Geometry check sheet. Reference: the model listing, model coordinates, mm. Face numbers are marked on the shaded views. A direction names the side the tool comes from. Give positions to 0.01 mm unless a question says otherwise; leave off trailing zeros. Write each loop counter-clockwise with the first axis right and the second up, starting at its lowest first coordinate (ties: lowest second). Pieces come first, ordered by that corner, then holes. Notation, with made-up numbers: M 58.25,74.25 L 62.25,74.25 A26 cw 62.25,102.25 Z; hole C 62.5,27 d6. An arc over 180 degrees is marked long. One line per item, written item: value. Start each with the question number.
1. Cross-section at B-B on x = 1.75. Record the cut outline in (y, z), then the cut area to 3 significant figures.
2. Gauge pin test, flat ends, axial feed: pin 1 (1.6 mm diameter, centred on x = -9, z = 4, fed in from +Y); pin 2 (4 mm diameter, centred on x = 9, y = -7, fed in from +Z); pin 3 (2 mm diameter, centred on x = 0, z = 21, fed in from +Y). Record the tip position at first contact, or that the pin passes through.
3. Tool access check on the marked faces 4, 5 and 6. Record the directions out of +Z, -Z, +X, -X, +Y, -Y that give a thin tool (end or side, any length) a straight path to the whole face; none if there is none.
4. Cross-section at C-C on y = -4. Record the cut outline in (x, z).
5. Scan lines: line 1 (Y direction, x = 0, z = 1.4); line 2 (X direction, y = -5, z = 8.5); line 3 (Y direction, x = 4.25, z = 15.5). Record each from-to range of solid material in increasing order.
6. Release check for a two-part mould opening along X. For the marked faces 1, 2 and 3 record: pulls with the +X half, pulls with the -X half, needs draft (parallel to the pull), parting line crosses it, or undercut.
7. Cross-section at A-A on z = 9. Record the cut outline in (x, y).
8. Cross-section at D-D on z = 4. Count the separate pieces of the cut face and the enclosed holes in it, then the cut area to 3 significant figures.
from build123d import *

# Parameters (mm, degrees)
BOSS_EXTRUDE1_DEPTH = 3
SKETCH2_W           = 13
SKETCH2_H           = 15
BOSS_EXTRUDE2_DEPTH = 27.5
SKETCH3_W           = 10.6
SKETCH3_H           = 13
CUT_EXTRUDE1_DEPTH  = 26.5
CUT_EXTRUDE2_DEPTH  = 31.5
SKETCH5_W           = 1.5
SKETCH5_H           = 27.57988307
CUT_EXTRUDE3_DEPTH  = 4
BOSS_EXTRUDE4_DEPTH = 2
FILLET2_R           = 1.5
FILLET3_R           = 1.5
SKETCH7_R           = 1
CUT_EXTRUDE4_DEPTH  = 4


with BuildPart() as part:
    # Sketch1 → Boss-Extrude1 (new body)
    with BuildSketch(Plane.XY):
        with BuildLine():
            Line((8.035256759, -13.057292233), (-7.964743241, -13.057292233))
            Line((-7.964743241, -13.057292233), (-7.964743241, 12.942707767))
            ThreePointArc((-7.964743241, 12.942707767), (-0.020633322, 16.942707767), (8.035256759, 13.172891138))
            Line((8.035256759, 13.172891138), (8.035256759, -13.057292233))
        make_face()
    extrude(amount=BOSS_EXTRUDE1_DEPTH)

    # Sketch2 → Boss-Extrude2 (add)
    with BuildSketch(Plane.XY.offset(3)):
        with Locations((0.035256759, -5.557292233)):
            Rectangle(SKETCH2_W, SKETCH2_H)
    extrude(amount=BOSS_EXTRUDE2_DEPTH)

    # Sketch3 → Cut-Extrude1 (cut, symmetric)
    with BuildSketch(Plane.XY.offset(3)):
        with Locations((-0.014743241, -5.807292233)):
            Rectangle(SKETCH3_W, SKETCH3_H)
    extrude(amount=CUT_EXTRUDE1_DEPTH, both=True, mode=Mode.SUBTRACT)

    # Sketch4 → Cut-Extrude2 (cut, through all)
    with BuildSketch(Plane.XY.offset(30.5)):
        with BuildLine():
            Line((-2.5, -8.94154935), (-2.5, -2.55973464))
            ThreePointArc((-2.5, -2.55973464), (0, -0.05973464), (2.5, -2.55973464))
            Line((2.5, -2.55973464), (2.5, -8.94154935))
            ThreePointArc((2.5, -8.94154935), (0, -11.44154935), (-2.5, -8.94154935))
        make_face()
    extrude(amount=-CUT_EXTRUDE2_DEPTH, mode=Mode.SUBTRACT)

    # Sketch5 → Cut-Extrude3 (cut, through all)
    with BuildSketch(Plane.XY.offset(3)):
        with Locations((-7.214743241, 0.732649302)):
            Rectangle(SKETCH5_W, SKETCH5_H)
        with Locations((7.285256759, 0.732649302)):
            Rectangle(SKETCH5_W, SKETCH5_H)
    extrude(amount=-CUT_EXTRUDE3_DEPTH, mode=Mode.SUBTRACT)

    # Sketch6 → Boss-Extrude4 (add)
    with BuildSketch(Plane.XY.offset(3)):
        Polygon((-6.464743241, -3.398686813), (-9.964743241, -3.398686813), (-9.964743241, -7.898686813), (-6.464743241, -7.898686813), (-6.464743241, -9.398686813), (-11.464743241, -9.398686813), (-11.464743241, -1.898686813), (-6.464743241, -1.898686813), align=None)
        Polygon((6.535256759, -3.398686813), (6.535256759, -1.898686813), (11.535256759, -1.898686813), (11.535256759, -9.398686813), (6.535256759, -9.398686813), (6.535256759, -7.898686813), (10.035256759, -7.898686813), (10.035256759, -3.398686813), align=None)
    extrude(amount=BOSS_EXTRUDE4_DEPTH)

    # Fillet2
    fillet2_edges = [part.edges().sort_by_distance(p)[0] for p in [
        (-9.964743241, -3.398686813, 4),
        (-11.464743241, -1.898686813, 4),
        (-11.464743241, -9.398686813, 4),
        (-9.964743241, -7.898686813, 4),
    ]]
    fillet(fillet2_edges, radius=FILLET2_R)

    # Fillet3
    fillet3_edges = [part.edges().sort_by_distance(p)[0] for p in [
        (10.035256759, -3.398686813, 4),
        (10.035256759, -7.898686813, 4),
        (11.535256759, -9.398686813, 4),
        (11.535256759, -1.898686813, 4),
    ]]
    fillet(fillet3_edges, radius=FILLET3_R)

    # Sketch7 → Cut-Extrude4 (cut, through all)
    with BuildSketch(Plane.XY.offset(3)):
        with Locations((0, 14.234326683)):
            Circle(SKETCH7_R)
        with Locations((0, 5.748094445)):
            Circle(SKETCH7_R)
    extrude(amount=-CUT_EXTRUDE4_DEPTH, mode=Mode.SUBTRACT)


solid = part.part
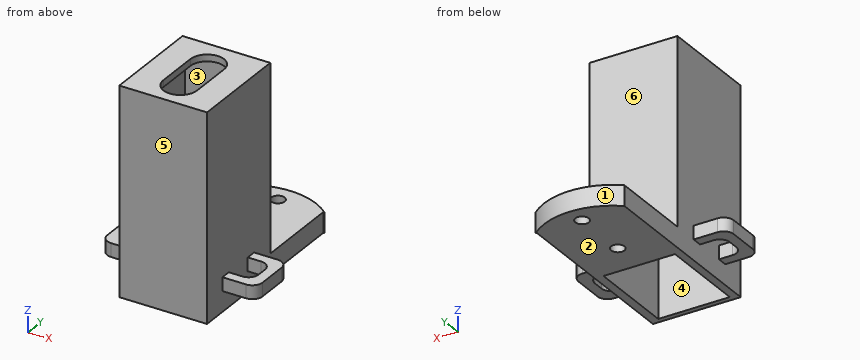
Report:
1. outline: M -13.06,0 L -12.31,0 L -12.31,29.5 L -10.73,29.5 L -10.73,30.5 L -13.06,30.5 Z; M -0.77,29.5 L 0.69,29.5 L 0.69,0 L 16.81,0 L 16.81,3 L 1.94,3 L 1.94,30.5 L -0.77,30.5 Z
1. area: 109 mm^2
2. pin 1: stops at y = -1.9
2. pin 2: stops at z = 5
2. pin 3: stops at y = 1.94
3. face 4: -Z
3. face 5: +Z, -Z, +X, -X, -Y
3. face 6: +Z, +X, -X, +Y
4. outline: M -11.46,3 L -9.67,3 L -9.67,5 L -11.46,5 Z; M -6.46,0 L -5.31,0 L -5.31,29.5 L -2.5,29.5 L -2.5,30.5 L -6.46,30.5 Z; M 2.5,29.5 L 5.29,29.5 L 5.29,0 L 6.54,0 L 6.54,30.5 L 2.5,30.5 Z; M 9.74,3 L 11.54,3 L 11.54,5 L 9.74,5 Z
5. line 1: y = -13.06 to -12.31, 0.69 to 4.75, 6.75 to 13.23, 15.23 to 16.94
5. line 2: x = -6.46 to -5.31, 5.29 to 6.54
5. line 3: y = -13.06 to -12.31, 0.69 to 1.94
6. face 1: parting line crosses it
6. face 2: needs draft
6. face 3: undercut
7. outline: M -6.46,-13.06 L 6.54,-13.06 L 6.54,1.94 L -6.46,1.94 Z; hole M -5.31,-12.31 L 5.29,-12.31 L 5.29,0.69 L -5.31,0.69 Z
8. separate pieces: 1
8. enclosed holes: 3
8. area: 101 mm^2
